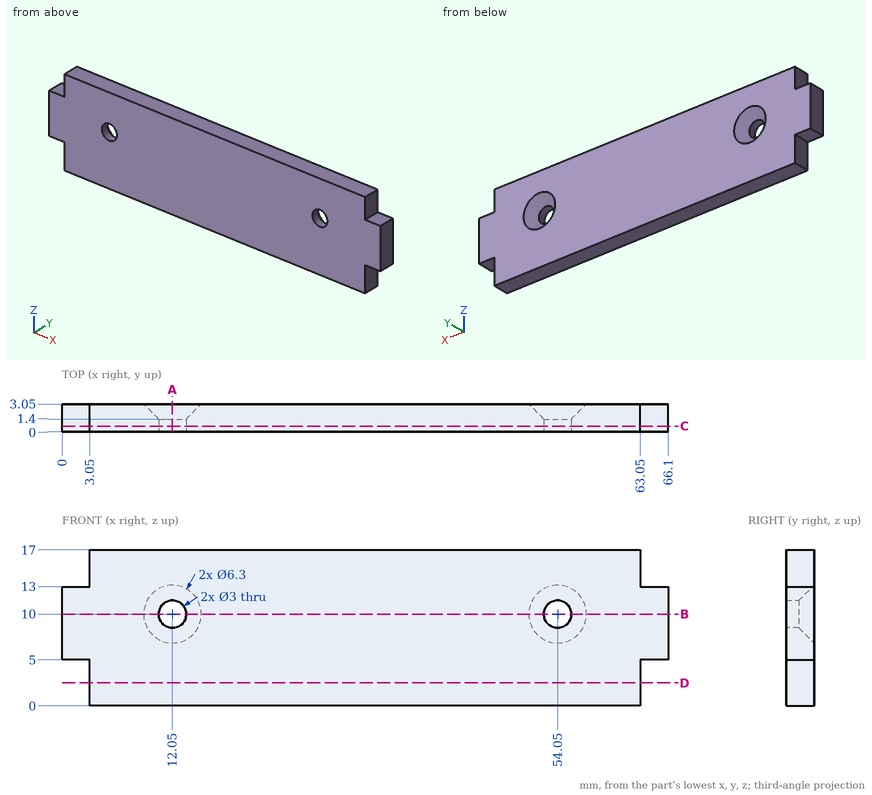
The drawing under review shows one solid part. Ordinate dimensions are in mm from its lowest x, y, z. Coordinates: 2 decimals unless noted, no trailing zeros. Loops run counter-clockwise (first coordinate to the right, second up) from the corner with the lowest first, then second, coordinate; pieces in that order, holes last. Notation, with made-up numbers: M 51.25,4 L 61.25,4 A7 ccw 61.25,12 Z; hole C 58,32.5 d8. An arc over 180 degrees is marked long. Use one line per item in the form item = value.
(1) Clearance check with flat-ended pins moving along their axes: P1, Ø0.9, axis at x = 64.5, y = 1, coming from the -Z side; P2, Ø1.5, axis at y = 1.5, z = 3.5, coming from the +X side; P3, Ø0.9, axis at x = 1.5, y = 2, coming from the +Z side. State where each tip first meets the part, or that it passes through.
Return value:
P1 = 5
P2 = 63.05
P3 = 13
(2) Consider section B-B (z = 10). Write out the cut boundary in (x, y).
Return value:
outline = M 0,0 L 10.55,0 L 10.55,1.4 L 8.9,3.05 L 0,3.05 Z; M 13.55,0 L 52.55,0 L 52.55,1.4 L 50.9,3.05 L 15.2,3.05 L 13.55,1.4 Z; M 55.55,0 L 66.1,0 L 66.1,3.05 L 57.2,3.05 L 55.55,1.4 Z
(3) Consider section D-D (z = 2.5). Write out the cut boundary in (x, y), and give its area (3 significant figures).
Return value:
outline = M 3.05,0 L 63.05,0 L 63.05,3.05 L 3.05,3.05 Z
area = 183 mm2
(4) Consider section A-A (x = 12.05). Write out the cut boundary in (y, z).
Return value:
outline = M 0,0 L 3.05,0 L 3.05,6.85 L 1.4,8.5 L 0,8.5 Z; M 0,11.5 L 1.4,11.5 L 3.05,13.15 L 3.05,17 L 0,17 Z
(5) Consider section C-C (y = 0.65). Write out the cut boundary in (x, z), and give its area (3 significant figures).
Return value:
outline = M 0,5 L 3.05,5 L 3.05,0 L 63.05,0 L 63.05,5 L 66.1,5 L 66.1,13 L 63.05,13 L 63.05,17 L 3.05,17 L 3.05,13 L 0,13 Z; hole C 12.05,10 d3; hole C 54.05,10 d3
area = 1,050 mm2
(6) For line 1 along X through (y, z) = (0.7, 10); line 2 along Z through (x, y) = (12.05, 0.5); line 3 along X through (y, z) = (2.55, 8.75), list the stretches that pass through material, from the lowest coordinate up. Write a range as from..to.
Return value:
line_1 = 0..10.55, 13.55..52.55, 55.55..66.1
line_2 = 0..8.5, 11.5..17
line_3 = 0..9.71, 14.39..51.71, 56.39..66.1
